Design review of the part built by this model. Coordinates are the model's own, in mm. Face numbers are marked on the shaded views. A direction names the side the tool comes from. Round coordinates to 2 decimals unless told otherwise and drop trailing zeros. Loops run counter-clockwise (first coordinate to the right, second up) from the corner with the lowest first, then second, coordinate; pieces in that order, holes last. Notation, with made-up numbers: M -11.75,-1 L 27.25,-1 A33 ccw 27.25,37 Z; hole C 11.25,44 d6. An arc over 180 degrees is marked long. Answer as CSV lines item,"result". Start each with the question number.
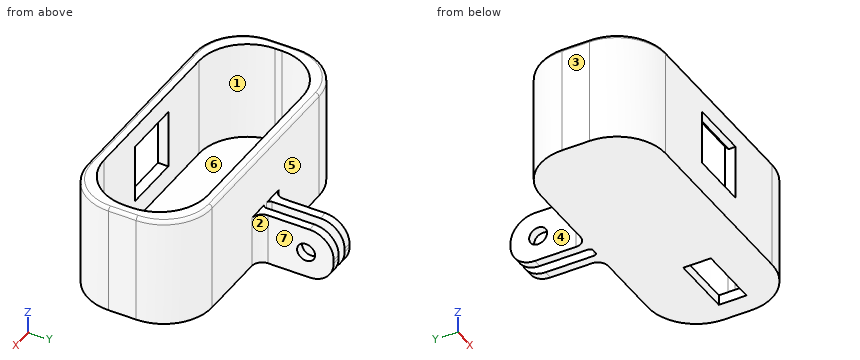
from build123d import *

# Parameters (mm, degrees)
SKETCH_W        = 82
SKETCH_H        = 36
PAD_DEPTH       = 32
SKETCH001_W     = 76
SKETCH001_H     = 30
POCKET_DEPTH    = 29
FILLET_R        = 14
SKETCH002_W     = 17
SKETCH002_H     = 16
POCKET001_DEPTH = 8
SKETCH003_W     = 18
SKETCH003_H     = 8
POCKET002_DEPTH = 5
SKETCH004_W     = 2.5
SKETCH004_H     = 15
PAD001_DEPTH    = 22
SKETCH005_R     = 2.6
POCKET003_DEPTH = 12
FILLET001_R     = 1
FILLET002_R     = 7
FILLET003_R     = 3
FILLET004_R     = 1
CHAMFER_SIZE    = 1


with BuildPart() as part:
    # Sketch → Pad (new body)
    with BuildSketch(Plane.XY):
        Rectangle(SKETCH_W, SKETCH_H)
    extrude(amount=PAD_DEPTH)

    # Sketch001 (on Face6 of Pad) → Pocket (cut)
    with BuildSketch(Plane.XY.offset(32)):
        Rectangle(SKETCH001_W, SKETCH001_H)
    extrude(amount=-POCKET_DEPTH, mode=Mode.SUBTRACT)

    # Fillet
    fillet_edges = [part.edges().sort_by_distance(p)[0] for p in [
        (-41, 18, 16),
        (-38, 15, 17.5),
        (-41, -18, 16),
        (-38, -15, 17.5),
        (41, 18, 16),
        (38, 15, 17.5),
        (41, -18, 16),
        (38, -15, 17.5),
    ]]
    fillet(fillet_edges, radius=FILLET_R)

    # Sketch002 → Pocket001 (cut)
    with BuildSketch(Plane(origin=(0, -15, 0), x_dir=(-1, 0, 0), z_dir=(0, 1, 0))):
        with Locations((0, 17)):
            Rectangle(SKETCH002_W, SKETCH002_H)
    extrude(amount=-POCKET001_DEPTH, mode=Mode.SUBTRACT)

    # Sketch003 (on Face2 of Pocket001) → Pocket002 (cut)
    with BuildSketch(Plane(origin=(0, 0, 0), x_dir=(1, 0, 0), z_dir=(0, 0, -1))):
        with Locations((26, 2)):
            Rectangle(SKETCH003_W, SKETCH003_H)
    extrude(amount=-POCKET002_DEPTH, mode=Mode.SUBTRACT)

    # Sketch004 (on Face1 of Pocket002) → Pad001 (join)
    with BuildSketch(Plane(origin=(0, 18, 0), x_dir=(-1, 0, 0), z_dir=(0, 1, 0))):
        with Locations((2.75, 7.5)):
            Rectangle(SKETCH004_W, SKETCH004_H)
        with Locations((-2.75, 7.5)):
            Rectangle(SKETCH004_W, SKETCH004_H)
    extrude(amount=PAD001_DEPTH)

    # Sketch005 (on Face8 of Pad001) → Pocket003 (cut)
    with BuildSketch(Plane.YZ.offset(4)):
        with Locations((32, 7.5)):
            Circle(SKETCH005_R)
    extrude(amount=-POCKET003_DEPTH, mode=Mode.SUBTRACT)

    # Fillet001
    fillet001_edges = [part.edges().sort_by_distance(p)[0] for p in [
        (-36.899495, 13.899495, 32),
        (-41, 0, 32),
        (-36.899495, -13.899495, 32),
        (0, -18, 32),
        (36.899495, -13.899495, 32),
        (41, 0, 32),
        (36.899495, 13.899495, 32),
        (0, 18, 32),
    ]]
    fillet(fillet001_edges, radius=FILLET001_R)

    # Fillet002
    fillet002_edges = [part.edges().sort_by_distance(p)[0] for p in [
        (-2.75, 40, 15),
        (2.75, 40, 15),
        (-2.75, 40, 0),
        (2.75, 40, 0),
    ]]
    fillet(fillet002_edges, radius=FILLET002_R)

    # Fillet003
    fillet003_edges = [part.edges().sort_by_distance(p)[0] for p in [
        (4, 18, 7.5),
        (-4, 18, 7.5),
    ]]
    fillet(fillet003_edges, radius=FILLET003_R)

    # Fillet004
    fillet004_edges = [part.edges().sort_by_distance(p)[0] for p in [
        (-1.5, 18, 7.5),
        (1.5, 18, 7.5),
    ]]
    fillet(fillet004_edges, radius=FILLET004_R)

    # Chamfer
    chamfer_edges = [part.edges().sort_by_distance(p)[0] for p in [
        (0, -15, 25),
    ]]
    chamfer(chamfer_edges, length=CHAMFER_SIZE)


solid = part.part
Item 1: To check wall thickness, follow line 1 (Y direction, x = -10, z = 8.5); line 2 (Z direction, x = 2.5, y = 32); line 3 (Z direction, x = 7, y = -2.5). State the ranges of each line that lie inside material, in increasing order.
Item 2: Insertion check: pin 1 Ø2 at (x, y) = (2, 28) entering from +Z; pin 2 Ø1.5 at (x, y) = (-20.5, 14) entering from +Z; pin 3 Ø7.5 at (y, z) = (34, 8) entering from -X. Each pin has a flat end and moves straight along its axis. Give the tip position at first contact, or say it passes through.
Item 3: Consider section A-A, the plane y = 32. Write out the cut boundary in (x, z).
Item 4: Tool access review of the marked faces 4, 5, 6 and 7: name each direction out of +Z, -Z, +X, -X, +Y, -Y from which nothing blocks a thin tool from reaching the whole face with its end or side.
Item 5: Consider section C-C, the plane z = 22. Write out the cut boundary in (x, y), then the cut area to 3 significant figures.
Item 6: The part is to be moulded in two halves that separate along Y. For the marked faces 1, 2 and 3, say which applies: +Y half, -Y half, draft (parallel to the pull), parting line (faces both ways), or undercut.
Item 7: Consider section B-B, the plane z = 27.5. Write out the cut boundary in (x, y), then the cut area to 3 significant figures.
Found:
1,line 1,"y = -18 to -15, 15 to 18"
1,line 2,"z = 0 to 4.9, 10.1 to 15"
1,line 3,"z = 0 to 3"
2,pin 1,"stops at z = 15"
2,pin 2,"stops at z = 3"
2,pin 3,"stops at x = -4"
3,outline,"M -4,0 L -1.5,0 L -1.5,4.9 L -4,4.9 Z; M -4,10.1 L -1.5,10.1 L -1.5,15 L -4,15 Z; M 1.5,0 L 4,0 L 4,4.9 L 1.5,4.9 Z; M 1.5,10.1 L 4,10.1 L 4,15 L 1.5,15 Z"
4,face 4,"+Z, -Z, -X, +Y"
4,face 5,"+Z, +Y"
4,face 6,"+Z"
4,face 7,"+Z, -Z, +X, +Y"
5,outline,"M -41,-4 A14 ccw -27,-18 L -8.5,-18 L -8.5,-15 L -24,-15 A14 cw -38,-1 L -38,1 A14 cw -24,15 L 24,15 A14 cw 38,1 L 38,-1 A14 cw 24,-15 L 8.5,-15 L 8.5,-18 L 27,-18 A14 ccw 41,-4 L 41,4 A14 ccw 27,18 L -27,18 A14 ccw -41,4 Z"
5,area,"621 mm^2"
6,face 1,"undercut"
6,face 2,"+Y half"
6,face 3,"draft"
7,outline,"M -41,-4 A14 ccw -27,-18 L 27,-18 A14 ccw 41,-4 L 41,4 A14 ccw 27,18 L -27,18 A14 ccw -41,4 Z; hole M -38,-1 A14 ccw -24,-15 L 24,-15 A14 ccw 38,-1 L 38,1 A14 ccw 24,15 L -24,15 A14 ccw -38,1 Z"
7,area,"672 mm^2"
